from build123d import *

# Parameters (mm, degrees)
SKETCH2_R           = 2.5
BOSS_EXTRUDE1_DEPTH = 65
CUT_EXTRUDE1_START  = -25
CUT_EXTRUDE1_DEPTH  = 25
FILLET1_R           = 1
FILLET2_R           = 1


with BuildPart() as part:
    # Sketch2 → Boss-Extrude1 (new body)
    with BuildSketch(Plane(origin=(0, 0, 0), x_dir=(1, 0, 0), z_dir=(0, 1, 0))):
        with Locations(Location((0.061061942, 0.061061942, 0), (0, 0, 270))):
            Circle(SKETCH2_R)
    extrude(amount=BOSS_EXTRUDE1_DEPTH)

    # Sketch3 → Cut-Extrude1 (cut)
    with BuildSketch(Plane(origin=(0, 65, 0), x_dir=(1, 0, 0), z_dir=(0, 1, 0)).offset(CUT_EXTRUDE1_START)):
        with BuildLine():
            Line((-1.00625914, 2.321775482), (1.173082806, 2.300126389))
            ThreePointArc((1.173082806, 2.300126389), (0.085895154, 2.560938601), (-1.00625914, 2.321775482))
        make_face()
    extrude(amount=CUT_EXTRUDE1_DEPTH, mode=Mode.SUBTRACT)

    # Fillet1
    # the kernel refuses this fillet: 1 mm, written as the material it takes off along each edge
    with BuildSketch(Plane(origin=(0.061061942, 65, -0.061061942), x_dir=(0.5312663336495629, 0, -0.8472048646759243), z_dir=(0.8472048646759243, 0, 0.5312663336495629))) as fillet1_piece_1:
        with BuildLine():
            CenterArc((2.5 - FILLET1_R, -FILLET1_R), FILLET1_R, 0, 90)
            Line((2.5 - FILLET1_R, 0), (2.5, 0))
            Line((2.5, 0), (2.5, -FILLET1_R))
        make_face()
    revolve(axis=Axis((0.061061942, 65, -0.061061942), (0, 1, 0)), revolution_arc=212.091055881, mode=Mode.SUBTRACT)
    with BuildSketch(Plane(origin=(0.061061942, 65, -0.061061942), x_dir=(0, 0, 1), z_dir=(-1, 0, 0))) as fillet1_piece_2:
        with BuildLine():
            CenterArc((2.5 - FILLET1_R, -FILLET1_R), FILLET1_R, 0, 90)
            Line((2.5 - FILLET1_R, 0), (2.5, 0))
            Line((2.5, 0), (2.5, -FILLET1_R))
        make_face()
    revolve(axis=Axis((0.061061942, 65, -0.061061942), (0, 1, 0)), revolution_arc=210.951767977, mode=Mode.SUBTRACT)

    # Fillet2
    fillet2_edges = [part.edges().sort_by_distance(p)[0] for p in [
        (0.061061942, 0, -2.561061942),
    ]]
    fillet(fillet2_edges, radius=FILLET2_R)


solid = part.part
Work out the finished part from the listing and answer in its coordinate system (mm). Round coordinates to 2 decimals unless told otherwise and drop trailing zeros. Loops run counter-clockwise (first coordinate to the right, second up) from the corner with the lowest first, then second, coordinate; pieces in that order, holes last. Notation, with made-up numbers: M 55,66.25 L 81,66.25 A18 ccw 81,101.25 Z; hole C -34.75,-15.5 d6. An arc over 180 degrees is marked long. One line per question, with ' | ' between items. Start each with the question number.
(1) A cutting plane is placed at A-A on y = 47. Write down the section's boundary in (x, z), plus the area to 3 significant figures.
(2) A cutting plane is placed at B-B on y = 27. Write down the section's boundary in (x, z), plus the area to 3 significant figures.
(3) Find the intervals of material crossed by line 1 (X direction, y = 10, z = 0.15); line 2 (Z direction, x = -0.2, y = 54.5); line 3 (Y direction, x = 1.7, z = 0.85), in increasing order.
Geometry check:
1) outline: M -1.01,-2.32 L 1.17,-2.3 A2.5 ccw long Z | area: 19.3 mm²
2) outline: C 0.06,-0.06 d5 | area: 19.6 mm²
3) line 1: x = -2.43 to 2.55 | line 2: z = -2.31 to 2.43 | line 3: y = 0.07 to 64.93
